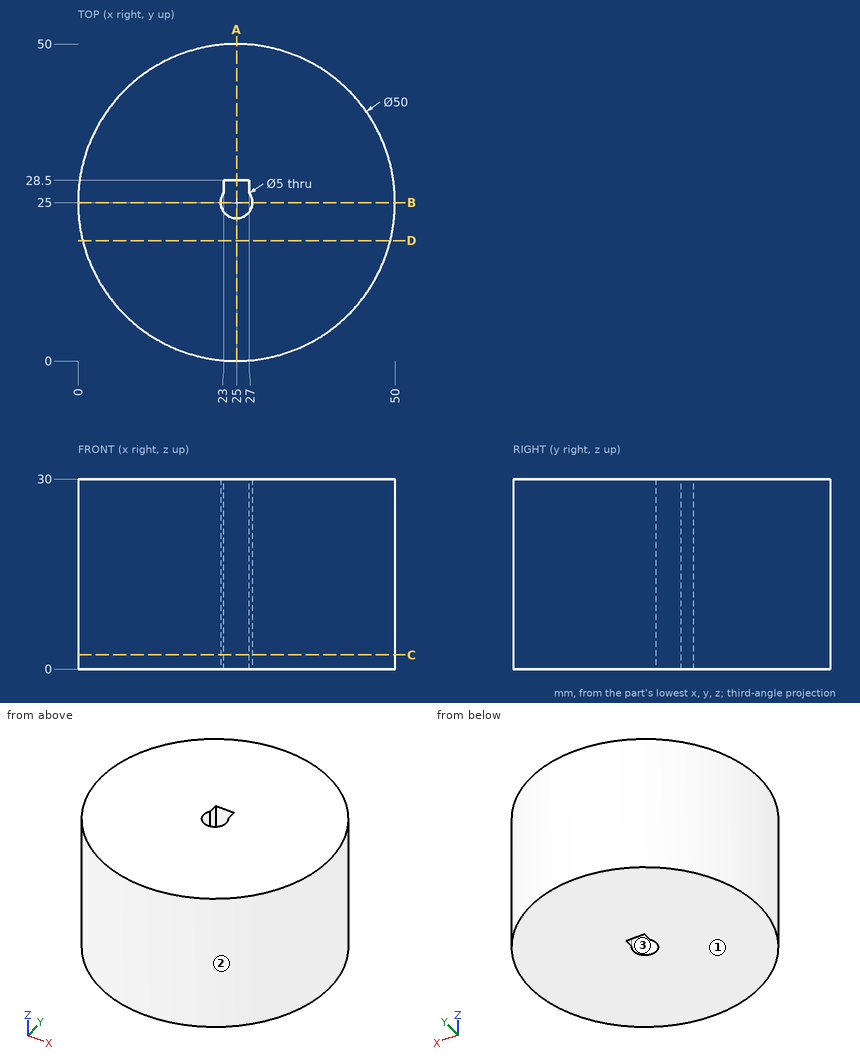
Job drawing, mm, ordinate dimensions from the low corner. One solid piece. Give positions to 0.01 mm unless a question says otherwise; leave off trailing zeros. Loops run counter-clockwise (first coordinate to the right, second up) from the corner with the lowest first, then second, coordinate; pieces in that order, holes last. Notation, with made-up numbers: M 74,16.25 L 91,16.25 A22 cw 91,50.25 Z; hole C 81.5,22 d10. An arc over 180 degrees is marked long. Use one line per item in the form item = value.
Item 1: Drill centre lines: L1, parallel to Y at x = 25, z = 8.75; L2, parallel to X at y = 24, z = 11; L3, parallel to Y at x = 44.5, z = 22. Where is each one in solid material? Low to high.
Filled in:
L1 = 0 to 22.5, 28.5 to 50
L2 = 0.02 to 22.71, 27.29 to 49.98
L3 = 9.36 to 40.64
Item 2: Flat gauge pins, fed straight in: pin 1 Ø3 at (x, y) = (25, 25) entering from +Z; pin 2 Ø1.5 at (x, z) = (32.5, 23.5) entering from +Y; pin 3 Ø1 at (y, z) = (27.5, 16.5) entering from +X; pin 4 Ø12 at (x, z) = (43.5, 19) entering from +Y. Where does each tip first touch, or does it go through?
Filled in:
pin_1 = through
pin_2 = 49.07
pin_3 = 49.92
pin_4 = 46.65
Item 3: Slice it at B-B on y = 25. List the corners of the cut face in (x, z), and give its area (3 significant figures).
Filled in:
outline = M 0,0 L 22.5,0 L 22.5,30 L 0,30 Z; M 27.5,0 L 50,0 L 50,30 L 27.5,30 Z
area = 1,350 mm^2
Item 4: Slice it at C-C on z = 2.25. List the corners of the cut face in (x, y), and give its area (3 significant figures).
Filled in:
outline = C 25,25 d50; hole M 23,26.5 A2.5 ccw long 27,26.5 L 27,28.5 L 23,28.5 Z
area = 1,940 mm^2
Item 5: Two-plate mould, pull along Y, no slides. Class the marked faces 1, 2 and 3: released by +Y, released by -Y, zero draft, split by the parting line, or undercut.
Filled in:
face_1 = zero draft
face_2 = split by the parting line
face_3 = undercut
Item 6: Slice it at A-A on x = 25. List the corners of the cut face in (y, z).
Filled in:
outline = M 0,0 L 22.5,0 L 22.5,30 L 0,30 Z; M 28.5,0 L 50,0 L 50,30 L 28.5,30 Z
Item 7: Slice it at D-D on y = 19. List the corners of the cut face in (x, z).
Filled in:
outline = M 0.73,0 L 49.27,0 L 49.27,30 L 0.73,30 Z
